For this review, use the dimensioned drawing (mm, ordinates from the lowest corner) and the shaded views. A direction names the side the tool comes from. Coordinates: 2 decimals unless noted, no trailing zeros. Order: outer loops, then holes, each group sorted by start corner. A loop starts at its lowest first (then second) coordinate and runs counter-clockwise, first axis right, second up. Notation, with made-up numbers: M 37.25,58 L 73.25,58 A36 ccw 73.25,96 Z; hole C 80,-32.5 d9. An arc over 180 degrees is marked long. Answer as CSV lines item,"result". Start each with the question number.
Q1. For P1, Ø23.5, axis at x = 27.5, z = 70, coming from the +Y side; P2, Ø2.5, axis at x = 5.5, z = 135, coming from the +Y side, all flat-tipped, find the tip position at first contact; note any pin that passes through.
Q2. Consider section C-C on z = 115. Write out the cut boundary in (x, y), and give its area (3 significant figures).
Q3. Machinability: for the marked faces 1 and 2, which of the approach directions +Z, -Z, +X, -X, +Y, -Y give a long, thin tool a straight path to every point of the face, cutting with its end or side? Answer none if there is none.
Q4. Consider section A-A on y = 8.25. Write out the cut boundary in (x, z), and give its area (3 significant figures).
Q5. Consider section B-B on x = 27.5. Write out the cut boundary in (y, z).
Q6. Wall thickness on L1, parallel to Z at x = 72.5, y = 6.75; L2, parallel to X at y = 5.75, z = 34; L3, parallel to Z at x = 36.5, y = 12.25: over which ranges is each line inside the solid? List them lowest first. Write a range as [from, to].
Q7. Consider section D-D on z = 31.5. Write out the cut boundary in (x, y).
Q8. The part is to be moulded in two halves that separate along Z. For the marked faces 3, 4, 5 and 6, say which applies: +Z half, -Z half, draft (parallel to the pull), parting line (faces both ways), or undercut.
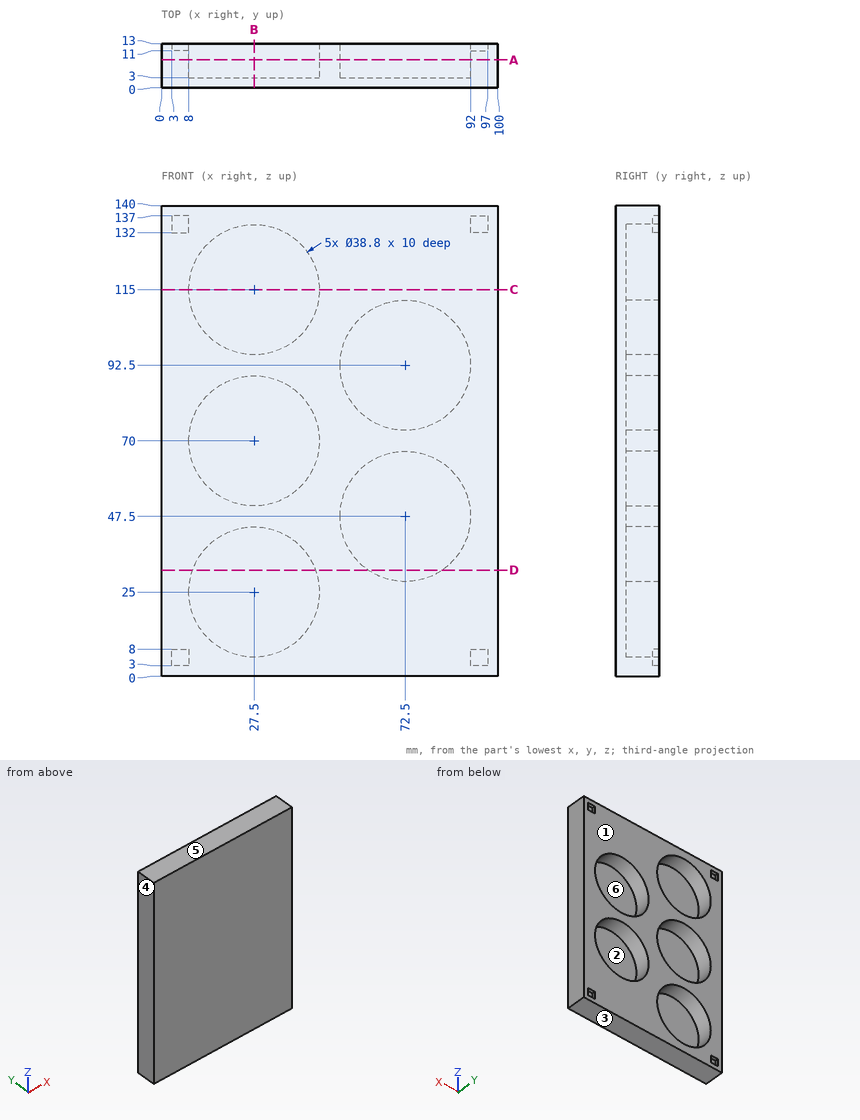
Evaluation:
1,P1,"stops at y = 3"
1,P2,"stops at y = 11"
2,outline,"M 0,0 L 100,0 L 100,13 L 46.9,13 L 46.9,3 L 8.1,3 L 8.1,13 L 0,13 Z"
2,area,"912 mm²"
3,face 1,"+Z, -Z, +X, -X, +Y"
3,face 2,"+Y"
4,outline,"M 0,0 L 100,0 L 100,140 L 0,140 Z; hole C 27.5,25 d38.8; hole C 27.5,70 d38.8; hole C 27.5,115 d38.8; hole C 72.5,47.5 d38.8; hole C 72.5,92.5 d38.8"
4,area,"8,090 mm²"
5,outline,"M 0,0 L 13,0 L 13,5.6 L 3,5.6 L 3,44.4 L 13,44.4 L 13,50.6 L 3,50.6 L 3,89.4 L 13,89.4 L 13,95.6 L 3,95.6 L 3,134.4 L 13,134.4 L 13,140 L 0,140 Z"
6,L1,"z = [0, 28.1], [66.9, 73.1], [111.9, 140]"
6,L2,"x = [0, 10.31], [44.69, 58.57], [86.43, 100]"
6,L3,"z = [0, 7.81], [42.19, 52.81], [87.19, 97.81], [132.19, 140]"
7,outline,"M 0,0 L 100,0 L 100,13 L 83.47,13 L 83.47,3 L 61.53,3 L 61.53,13 L 45.78,13 L 45.78,3 L 9.22,3 L 9.22,13 L 0,13 Z"
8,face 3,"-Z half"
8,face 4,"draft"
8,face 5,"+Z half"
8,face 6,"undercut"
